```python
from build123d import *

# Parameters (mm, degrees)
SKETCH1_W           = 8
SKETCH1_H           = 200
BOSS_EXTRUDE1_DEPTH = 2.5
SKETCH2_R           = 1.5
CUT_EXTRUDE1_DEPTH  = 196.656868011
CUT_EXTRUDE2_DEPTH  = 196.779493308


with BuildPart() as part:
    # Sketch1 → Boss-Extrude1 (new body)
    with BuildSketch(Plane(origin=(0, 0, 0), x_dir=(1, 0, 0), z_dir=(0, 1, 0))):
        with Locations((0, 95.6)):
            Rectangle(SKETCH1_W, SKETCH1_H)
    extrude(amount=BOSS_EXTRUDE1_DEPTH)

    # Sketch2 → Cut-Extrude1 (cut, through all)
    with BuildSketch(Plane(origin=(0, 2.5, 0), x_dir=(1, 0, 0), z_dir=(0, 1, 0))):
        with Locations(Location((0, 0.1, 0), (0, 0, 270))):
            Circle(SKETCH2_R)
        with Locations(Location((0, 10.1, 0), (0, 0, 270))):
            Circle(SKETCH2_R)
        with Locations(Location((0, 20.1, 0), (0, 0, 270))):
            Circle(SKETCH2_R)
        with Locations(Location((0, 30.1, 0), (0, 0, 270))):
            Circle(SKETCH2_R)
        with Locations(Location((0, 40.1, 0), (0, 0, 270))):
            Circle(SKETCH2_R)
        with Locations(Location((0, 50.1, 0), (0, 0, 270))):
            Circle(SKETCH2_R)
        with Locations(Location((0, 60.1, 0), (0, 0, 270))):
            Circle(SKETCH2_R)
        with Locations(Location((0, 70.1, 0), (0, 0, 270))):
            Circle(SKETCH2_R)
        with Locations(Location((0, 80.1, 0), (0, 0, 270))):
            Circle(SKETCH2_R)
        with Locations(Location((0, 90.1, 0), (0, 0, 270))):
            Circle(SKETCH2_R)
        with Locations(Location((0, 100.1, 0), (0, 0, 270))):
            Circle(SKETCH2_R)
        with Locations(Location((0, 110.1, 0), (0, 0, 270))):
            Circle(SKETCH2_R)
        with Locations(Location((0, 120.1, 0), (0, 0, 270))):
            Circle(SKETCH2_R)
        with Locations(Location((0, 130.1, 0), (0, 0, 270))):
            Circle(SKETCH2_R)
        with Locations(Location((0, 140.1, 0), (0, 0, 270))):
            Circle(SKETCH2_R)
        with Locations(Location((0, 150.1, 0), (0, 0, 270))):
            Circle(SKETCH2_R)
        with Locations(Location((0, 160.1, 0), (0, 0, 270))):
            Circle(SKETCH2_R)
        with Locations(Location((0, 170.1, 0), (0, 0, 270))):
            Circle(SKETCH2_R)
        with Locations(Location((0, 180.1, 0), (0, 0, 270))):
            Circle(SKETCH2_R)
        with Locations(Location((0, 190.1, 0), (0, 0, 270))):
            Circle(SKETCH2_R)
    extrude(amount=-CUT_EXTRUDE1_DEPTH, mode=Mode.SUBTRACT)

    # Sketch3 → Cut-Extrude2 (cut, through all)
    with BuildSketch(Plane(origin=(4, 0, 0), x_dir=(0, 0, -1), z_dir=(1, 0, 0))):
        Polygon((26.1, 2.5), (24.1, 2.5), (25.1, 2.1), align=None)
        Polygon((35.1, 0.4), (34.1, 0), (36.1, 0), align=None)
        Polygon((45.1, 0.4), (44.1, 0), (46.1, 0), align=None)
        Polygon((55.1, 0.4), (54.1, 0), (56.1, 0), align=None)
        Polygon((6.1, 2.5), (4.1, 2.5), (5.1, 2.1), align=None)
        Polygon((16.1, 2.5), (14.1, 2.5), (15.1, 2.1), align=None)
        Polygon((15.1, 0.4), (16.1, 0), (14.1, 0), align=None)
        Polygon((25.1, 0.4), (26.1, 0), (24.1, 0), align=None)
        Polygon((36.1, 2.5), (34.1, 2.5), (35.1, 2.1), align=None)
        Polygon((46.1, 2.5), (44.1, 2.5), (45.1, 2.1), align=None)
        Polygon((56.1, 2.5), (54.1, 2.5), (55.1, 2.1), align=None)
        Polygon((64.1, 2.5), (65.1, 2.1), (66.1, 2.5), align=None)
        Polygon((66.1, 0), (64.1, 0), (65.1, 0.4), align=None)
        Polygon((76.1, 2.5), (74.1, 2.5), (75.1, 2.1), align=None)
        Polygon((75.1, 0.4), (76.1, 0), (74.1, 0), align=None)
        Polygon((86.1, 2.5), (84.1, 2.5), (85.1, 2.1), align=None)
        Polygon((85.1, 0.4), (86.1, 0), (84.1, 0), align=None)
        Polygon((96.1, 2.5), (94.1, 2.5), (95.1, 2.1), align=None)
        Polygon((95.1, 0.4), (96.1, 0), (94.1, 0), align=None)
        Polygon((106.1, 2.5), (104.1, 2.5), (105.1, 2.1), align=None)
        Polygon((105.1, 0.4), (106.1, 0), (104.1, 0), align=None)
        Polygon((116.1, 2.5), (114.1, 2.5), (115.1, 2.1), align=None)
        Polygon((115.1, 0.4), (116.1, 0), (114.1, 0), align=None)
        Polygon((126.1, 2.5), (124.1, 2.5), (125.1, 2.1), align=None)
        Polygon((125.1, 0.4), (126.1, 0), (124.1, 0), align=None)
        Polygon((136.1, 2.5), (134.1, 2.5), (135.1, 2.1), align=None)
        Polygon((135.1, 0.4), (136.1, 0), (134.1, 0), align=None)
        Polygon((146.1, 2.5), (144.1, 2.5), (145.1, 2.1), align=None)
        Polygon((145.1, 0.4), (146.1, 0), (144.1, 0), align=None)
        Polygon((156.1, 2.5), (154.1, 2.5), (155.1, 2.1), align=None)
        Polygon((155.1, 0.4), (156.1, 0), (154.1, 0), align=None)
        Polygon((166.1, 2.5), (164.1, 2.5), (165.1, 2.1), align=None)
        Polygon((166.1, 0), (164.1, 0), (165.1, 0.4), align=None)
        Polygon((176.1, 2.5), (174.1, 2.5), (175.1, 2.1), align=None)
        Polygon((175.1, 0.4), (176.1, 0), (174.1, 0), align=None)
        Polygon((186.1, 2.5), (184.1, 2.5), (185.1, 2.1), align=None)
        Polygon((185.1, 0.4), (186.1, 0), (184.1, 0), align=None)
    extrude(amount=-CUT_EXTRUDE2_DEPTH, mode=Mode.SUBTRACT)


solid = part.part
```
Could you check a few things on this model? Use its own coordinates, in mm. Coordinates: 2 decimals unless noted, no trailing zeros. Return JSON: item names as keys, results as strings.
(1) I'm going to push a flat-ended pin straight in: pin 1 (4 mm diameter, centred on x = 0, z = -90.1, fed in from +Y). Where does the tip first touch, or does it pass through?
Numbers:
{"pin 1": "stops at y = 2.5"}
(2) I need wall thicknesses on L1, parallel to X at y = 0.45, z = -50; L2, parallel to X at y = 1.1, z = -70.5; L3, parallel to Y at x = 0.5, z = -125. Which ranges of each line are inside material? Lowest first, please.
Numbers:
{"L1": "x = -4 to -1.5, 1.5 to 4", "L2": "x = -4 to -1.45, 1.45 to 4", "L3": "y = 0.36 to 2.14"}
(3) Imagine slicing it at A-A, the plane y = 0.85. Count the separate pieces of the cut face and the enclosed holes in it, then the cut area to 3 significant figures.
Numbers:
{"separate pieces": "1", "enclosed holes": "20", "area": "1,460 mm2"}
